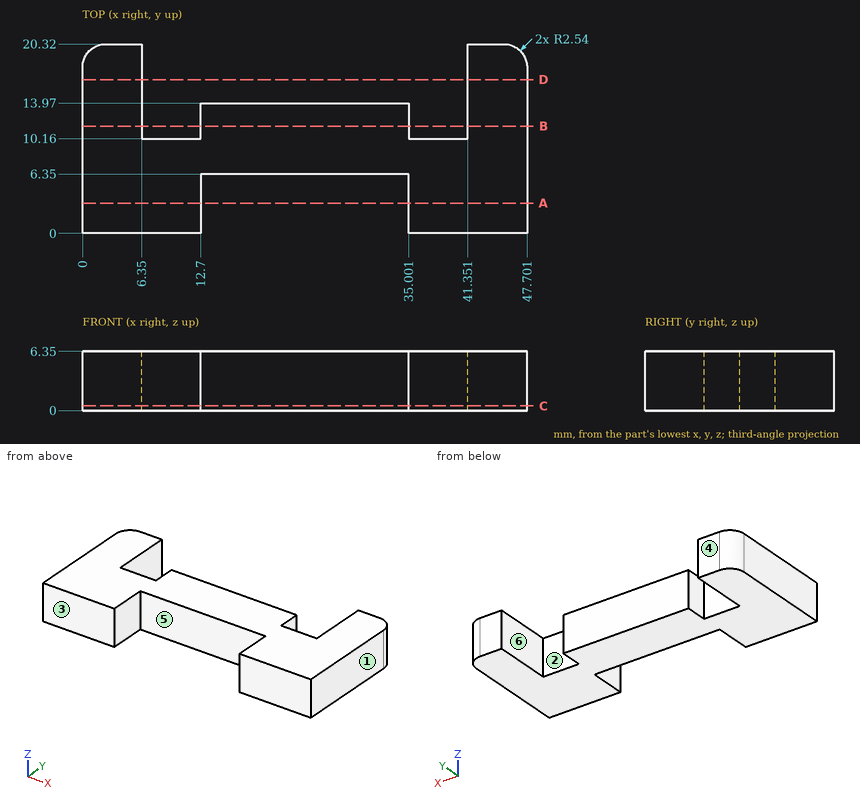
Geometry: see drawing. Coordinates: mm, zero at the bounding-box minimum. A direction names the side the tool comes from. Round coordinates to 2 decimals unless told otherwise and drop trailing zeros. Loops run counter-clockwise (first coordinate to the right, second up) from the corner with the lowest first, then second, coordinate; pieces in that order, holes last. Notation, with made-up numbers: (-16.5, 61.5) - (8.5, 61.5) arc R14 ccw to (8.5, 81.5) - close; hole circle Ø4 at (19, -3.5). An arc over 180 degrees is marked (long way). Write item = value, one per line. Start each with the question number.
(1) Section query C-C, the plane z = 0.5. Output: boundary loops of the cut face in (x, y).
(2) Section query D-D, the plane y = 16.5. Output: boundary loops of the cut face in (x, z).
(3) Ray query, line 1 along X through (y, z) = (10.75, 5.75); line 2 along X through (y, z) = (14.5, 0.5); line 3 along X through (y, z) = (1.25, 3). Return the intervals inside material, ascending. Write a range as from..to.
(4) Section query B-B, the plane y = 11.5. Output: boundary loops of the cut face in (x, z).
(5) Pin query (flat end, axial travel): pin 1 (1 mm diameter, centred on x = 18.5, z = 4, fed in from -Y); pin 2 (2 mm diameter, centred on x = 29, y = 12, fed in from -Z); pin 3 (1 mm diameter, centred on x = 8, z = 1.5, fed in from +Y). Return the tip coordinate at first contact, or that it passes through.
(6) Pull-direction query (X, two-part tool) for the marked faces 1, 2 and 3; classes: +X half, -X half, draft (parallel to the pull), parting line (faces both ways), or undercut.
(7) Section query A-A, the plane y = 3.25. Output: boundary loops of the cut face in (x, z).
(8) Set-up query: the marked faces 4, 5 and 6. Return all of +Z, -Z, +X, -X, +Y, -Y with unobstructed straight access to the full face (end or side cutting, diameter ignored); none if empty.
Conclusion:
q1.outline = (0, 0) - (12.7, 0) - (12.7, 6.35) - (35, 6.35) - (35, 0) - (47.7, 0) - (47.7, 17.78) arc R2.54 ccw to (45.16, 20.32) - (41.35, 20.32) - (41.35, 10.16) - (35, 10.16) - (35, 13.97) - (12.7, 13.97) - (12.7, 10.16) - (6.35, 10.16) - (6.35, 20.32) - (2.54, 20.32) arc R2.54 ccw to (0, 17.78) - close
q2.outline = (0, 0) - (6.35, 0) - (6.35, 6.35) - (0, 6.35) - close; (41.35, 0) - (47.7, 0) - (47.7, 6.35) - (41.35, 6.35) - close
q3.line_1 = 0..6.35, 12.7..35, 41.35..47.7
q3.line_2 = 0..6.35, 41.35..47.7
q3.line_3 = 0..12.7, 35..47.7
q4.outline = (0, 0) - (6.35, 0) - (6.35, 6.35) - (0, 6.35) - close; (12.7, 0) - (35, 0) - (35, 6.35) - (12.7, 6.35) - close; (41.35, 0) - (47.7, 0) - (47.7, 6.35) - (41.35, 6.35) - close
q5.pin_1 = 6.35
q5.pin_2 = 0
q5.pin_3 = 10.16
q6.face_1 = +X half
q6.face_2 = undercut
q6.face_3 = draft
q7.outline = (0, 0) - (12.7, 0) - (12.7, 6.35) - (0, 6.35) - close; (35, 0) - (47.7, 0) - (47.7, 6.35) - (35, 6.35) - close
q8.face_4 = +Z, -Z, +X, -X, +Y
q8.face_5 = +Z, -Z, -Y
q8.face_6 = +Z, -Z, +Y
